Autodesk Inventor part; units mm, degrees
ref_plane "YZ Plane" through (0, 0, 0) normal (1, 0, 0) x (0, 1, 0)
ref_plane "XZ Plane" through (0, 0, 0) normal (0, 1, 0) x (-1, 0, 0)
ref_plane "XY Plane" through (0, 0, 0) normal (0, 0, 1) x (1, 0, 0)
sketch "Sketch1" plane through (0, 0, 0) normal (0, 1, 0) x (-1, 0, 0)
  line L0 (0, 0) -> (0, -150)
  line L1 (0, -150) -> (50, -150)
  line L2 (0, 0) -> (50, -44.9152) construction
  line L3 (50, -44.9152) -> (50, -150) construction
  spline S0 degree 2 poles (0, 0) (50, -44.9152) (50, -150) knots 1 1 1 2 2 2
  dimension "d0" = 150
  dimension "d2" = 50
extrude "Extrusion7" add sketch "Sketch1" along normal blind 150
sketch "Sketch5" plane through (0, 0, -150) normal (0, 0, -1) x (-1, 0, 0)
  line L0 (0, 0) -> (0, 150)
  line L1 (0, 0) -> (20, 0)
  line L2 (0, 0) -> (50, 0)
  line L3 (20, 0) -> (20, 75)
  line L4 (25, 80) -> (15, 80)
  line L5 (15, 80) -> (15, 70)
  line L6 (15, 70) -> (25, 70)
  line L7 (25, 70) -> (25, 80)
  line L8 (25, 80) -> (15, 70) construction
  line L9 (15, 80) -> (25, 70) construction
  dimension "d57" = 20
  dimension "d58" = 75
  dimension "d59" = 10
  dimension "d60" = 10
extrude "Extrusion8" add sketch "Sketch5" along normal blind 10
sketch "Sketch6" plane through (0, 0, 0) normal (0, -1, 0) x (1, 0, 0)
  line L0 (0, 0) -> (0, -150)
  line L1 (0, -150) -> (-20, -150)
  line L2 (0, -150) -> (-50, -150)
  line L3 (-20, -150) -> (-20, -100)
  line L4 (-25.15, -105.15) -> (-14.85, -105.15)
  line L5 (-14.85, -105.15) -> (-14.85, -94.85)
  line L6 (-14.85, -94.85) -> (-25.15, -94.85)
  line L7 (-25.15, -94.85) -> (-25.15, -105.15)
  line L8 (-25.15, -105.15) -> (-14.85, -94.85) construction
  line L9 (-14.85, -105.15) -> (-25.15, -94.85) construction
  dimension "d51" = 20
  dimension "d52" = 50
  dimension "d53" = 10.3
  dimension "d54" = 10.3
extrude "Extrusion9" cut sketch "Sketch6" against normal blind 10
sketch "Sketch7" plane through (0, 150, 0) normal (0, 1, 0) x (1, 0, 0)
  line L0 (0, 150) -> (-50, 150)
  line L1 (0, 150) -> (-20, 150)
  line L2 (-20, 150) -> (-20, 100)
  line L3 (-15, 95) -> (-25, 95)
  line L4 (-25, 95) -> (-25, 105)
  line L5 (-25, 105) -> (-15, 105)
  line L6 (-15, 105) -> (-15, 95)
  line L7 (-15, 95) -> (-25, 105) construction
  line L8 (-25, 95) -> (-15, 105) construction
  point P0 (0, 0)
  dimension "d61" = 20
  dimension "d62" = 50
  dimension "d63" = 10
  dimension "d64" = 10
extrude "Extrusion10" add sketch "Sketch7" along normal blind 10
sketch "Sketch8" plane through (0, 0, 0) normal (1, 0, 0) x (0, 0, -1)
  line L0 (0, 0) -> (0, 150)
  line L1 (0, 75) -> (75, 75) construction
  line L2 (0, 150) -> (150, 150)
  circle A0 centre (75, 75) radius 6.25
  line L3 (75, 75) -> (86, 75)
  line L4 (75, 75) -> (80.5, 84.5263)
  line L5 (75, 75) -> (69.5, 84.5263)
  line L6 (75, 75) -> (64, 75)
  line L7 (75, 75) -> (69.5, 65.4737)
  line L8 (75, 75) -> (80.5, 65.4737)
  line L9 (80.5, 65.4737) -> (86, 75)
  line L10 (80.5, 84.5263) -> (86, 75)
  line L11 (69.5, 84.5263) -> (80.5, 84.5263)
  line L12 (69.5, 84.5263) -> (64, 75)
  line L13 (64, 75) -> (69.5, 65.4737)
  line L14 (80.5, 65.4737) -> (69.5, 65.4737)
  dimension "d67" = 75
  dimension "d69" = 12.5
  dimension "d70" = 11
  dimension "d73" = 360
extrude "Extrusion11" cut sketch "Sketch8" against normal blind 100
extrude "Extrusion12" add sketch "Sketch8" against normal blind 5 contours L3 L9 L8 A0 | A0 L4 L10 L3 | A0 L5 L11 L4 | L8 L14 L7 A0 | A0 L6 L12 L5 | L7 L13 L6 A0
properties part number "3DPrintShapeCorner"
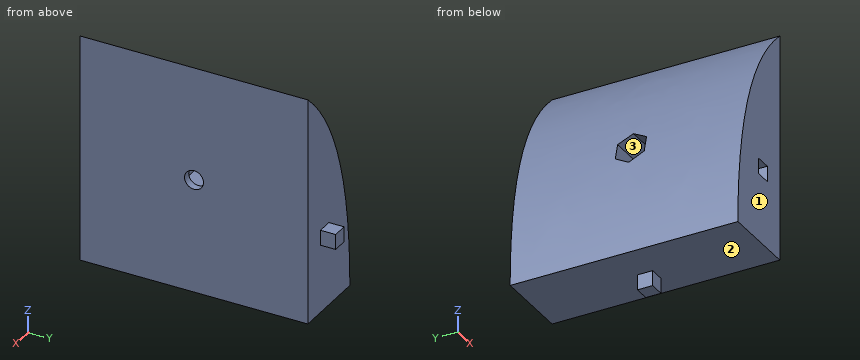
Here's how the part is built. I have some questions about the finished solid (model axes, mm). Face numbers are marked on the shaded views. Coordinates: 2 decimals unless noted, no trailing zeros.
1) Will these pins go through, and if not, where does the flat tip stop? pin 1 (3.5 mm diameter, centred on x = -25, z = -75.5, fed in from -Y); pin 2 (8 mm diameter, centred on x = -20.5, z = -154.5, fed in from +Y); pin 3 (5 mm diameter, centred on x = -20.5, y = 153.5, fed in from -Z); pin 4 (8 mm diameter, centred on x = -12.5, y = 25, fed in from -Z).
2) I need wall thicknesses on line 1 (Y direction, x = -1.1, z = -75); line 2 (Y direction, x = -3, z = -51); line 3 (Z direction, x = -1.2, y = 75). Which ranges of each line are inside material? Lowest first, please.
3) We'd pull the mould along Y, two halves only. Please class the marked faces 1, 2 and 3: +Y half, -Y half, draft (parallel to the pull), parting line (faces both ways), or undercut.
Response values:
1. pin 1: stops at y = 0
1. pin 2: stops at y = 80
1. pin 3: stops at z = -105
1. pin 4: stops at z = -150
2. line 1: y = 0 to 68.75, 81.25 to 150
2. line 2: y = 0 to 150
2. line 3: z = -150 to -81.25, -68.75 to -1.09
3. face 1: -Y half
3. face 2: draft
3. face 3: undercut
